Read the model definition and answer for the solid it produces. Units are mm, in the model's axes. A direction names the side the tool comes from. Give positions to 0.01 mm unless a question says otherwise; leave off trailing zeros. Order: outer loops, then holes, each group sorted by start corner. A loop starts at its lowest first (then second) coordinate and runs counter-clockwise, first axis right, second up. Notation, with made-up numbers: (-3, 26) - (55, 26) arc R24 cw to (55, 46) - close; hole circle Ø3 at (14, 81). An arc over 180 degrees is marked (long way). Use a Markdown table: item, result. Add a question column.
1. Flat-ended cylindrical pins translate along their axes: P1, Ø0.6, axis at x = 0, y = -3, coming from the +Z side; P2, Ø1, axis at x = 4.5, y = 0.5, coming from the -Z side. Find the tip coordinate at first contact, or state that the pin passes through.
2. Which of the six approach directions +Z, -Z, +X, -X, +Y, -Y give full straight-line access (tool end or side, diameter ignored) to faces 4 (the flat face through (-6.5, 0, 3)), 5 (the flat face through (0, 0, 0)), 6 (the flat face through (0, 3, 2.5)), 7 (the flat face through (-4.5, 0, 3)), 8 (the flat face through (5.131, -0.056, 4.986))?
3. For a pull along Y with two mould halves and no side action, classify faces 1 (the flat face through (0, -3, 2.5)), 2 (the flat face through (4.5, 0, 3)), 3 (the flat face through (0, -4, 2)) as released by +Y, released by -Y, zero draft, split by the parting line, or undercut.
4. Consider L1, parallel to X at y = 1.5, z = 2.75; L2, parallel to Y at x = -3, z = 2.4; L3, parallel to Z at x = -1, y = -1.25. Determine where each line is inside the solid, lowest interval first.
5. A cutting plane is placed at D-D on x = 2.25. Determine the outline of the cut face in (y, z), and give its area (3 significant figures).
6. A cutting plane is placed at C-C on y = -1.75. Determine the outline of the cut face in (x, z).
7. A cutting plane is placed at A-A on z = 2.2. Determine the outline of the cut face in (x, y), and give its area (3 significant figures).
8. A cutting plane is placed at B-B on z = 4.4. Determine the outline of the cut face in (x, y).
```python
from build123d import *

# Parameters (mm, degrees)
F0_W     = 13
F0_H     = 8
F3_DEPTH = 2
F1_W     = 13
F1_H     = 8
F1_W_2   = 9
F1_H_2   = 4
F4_DEPTH = 4
F5_START = 2.5
F2_W     = 9
F2_H     = 2
F5_DEPTH = 1.5
F6_W     = 2.7
F6_H     = 8
F7_DEPTH = 2
F9_DEPTH = 8.001


with BuildPart() as f3:
    # F0 (on Top) → F3 (new body)
    with BuildSketch(Plane.XY):
        Rectangle(F0_W, F0_H)
    extrude(amount=F3_DEPTH)

    # F1 (on Top) → F4 (join)
    with BuildSketch(Plane.XY):
        Rectangle(F1_W, F1_H)
        Rectangle(F1_W_2, F1_H_2, mode=Mode.SUBTRACT)
    extrude(amount=F4_DEPTH)

    # F2 (on Top) → F5 (cut)
    with BuildSketch(Plane.XY.offset(F5_START)):
        with Locations((0, 3)):
            Rectangle(F2_W, F2_H)
        with Locations((0, -3)):
            Rectangle(F2_W, F2_H)
    extrude(amount=F5_DEPTH, mode=Mode.SUBTRACT)

    # F6 (on face) → F7 (join)
    with BuildSketch(Plane.XY.offset(4)):
        with Locations((-5.15, 0)):
            Rectangle(F6_W, F6_H)
        with Locations((5.15, 0)):
            Rectangle(F6_W, F6_H)
    extrude(amount=F7_DEPTH)

    # F8 (on face) → F9 (cut, through all)
    with BuildSketch(Plane.XZ.offset(4)):
        Polygon((-3.8, 6), (-6.5, 6), (-3.8, 4), align=None)
        Polygon((3.8, 4), (6.5, 6), (3.8, 6), align=None)
    extrude(amount=-F9_DEPTH, mode=Mode.SUBTRACT)


solid = f3.part
```
Output values:
| question | item | result |
|---|---|---|
| 1 | P1 | z = 2.5 |
| 1 | P2 | z = 0 |
| 2 | face 4 | +Z, -Z, -X, +Y, -Y |
| 2 | face 5 | -Z, +X, -X, +Y, -Y |
| 2 | face 6 | +Y, -Y |
| 2 | face 7 | none |
| 2 | face 8 | +Z, +Y, -Y |
| 3 | face 1 | zero draft |
| 3 | face 2 | undercut |
| 3 | face 3 | released by -Y |
| 4 | L1 | -6.5 to -4.5, 4.5 to 6.5 |
| 4 | L2 | -4 to -2, 2 to 4 |
| 4 | L3 | 0 to 2 |
| 5 | outline | (-4, 0) - (4, 0) - (4, 2.5) - (2, 2.5) - (2, 2) - (-2, 2) - (-2, 2.5) - (-4, 2.5) - close |
| 5 | area | 18.0 mm² |
| 6 | outline | (-6.5, 0) - (6.5, 0) - (6.5, 6) - (3.8, 4) - (4.5, 4) - (4.5, 2) - (-4.5, 2) - (-4.5, 4) - (-3.8, 4) - (-6.5, 6) - close |
| 7 | outline | (-6.5, -4) - (6.5, -4) - (6.5, 4) - (-6.5, 4) - close; hole (-4.5, -2) - (4.5, -2) - (4.5, 2) - (-4.5, 2) - close |
| 7 | area | 68.0 mm² |
| 8 | outline | (-6.5, -4) - (-4.34, -4) - (-4.34, 4) - (-6.5, 4) - close; (4.34, -4) - (6.5, -4) - (6.5, 4) - (4.34, 4) - close |
